```python
from build123d import *

# Parameters (mm, degrees)
BOSS_EXTRUDE1_DEPTH      = 2.38125
BOSS_EXTRUDE1_DEPTH_BACK = 2.38125
SKETCH3_R                = 3.175
SKETCH3_R_2              = 1.4605
CHAMFER1_SIZE            = 0.17145
CUT_EXTRUDE1_DEPTH       = 6.082479863
CUT_EXTRUDE1_DEPTH_BACK  = 6.082479863
SKETCH4_R                = 1.6002


with BuildPart() as part:
    # Sketch3 → Boss-Extrude1 (new, two sides: drawn at the far end of the back side and taken through both)
    with BuildSketch(Plane.XY.offset(-BOSS_EXTRUDE1_DEPTH_BACK)):
        Circle(SKETCH3_R)
        Circle(SKETCH3_R_2, mode=Mode.SUBTRACT)
    extrude(amount=BOSS_EXTRUDE1_DEPTH + BOSS_EXTRUDE1_DEPTH_BACK)

    # Chamfer1
    chamfer1_edges = [part.edges().sort_by_distance(p)[0] for p in [
        (-3.175, 0, -2.38125),
        (-1.4605, 0, -2.38125),
        (-3.175, 0, 2.38125),
        (-1.4605, 0, 2.38125),
    ]]
    chamfer(chamfer1_edges, length=CHAMFER1_SIZE)

    # Sketch4 → Cut-Extrude1 (cut, two sides: drawn at the far end of the back side and taken through both)
    with BuildSketch(Plane.XY.offset(-CUT_EXTRUDE1_DEPTH_BACK)):
        Circle(SKETCH4_R)
    extrude(amount=CUT_EXTRUDE1_DEPTH + CUT_EXTRUDE1_DEPTH_BACK, mode=Mode.SUBTRACT)


solid = part.part
```
Here's how the part is built. I have some questions about the finished solid (model axes, mm). Round coordinates to 2 decimals unless told otherwise and drop trailing zeros. Order: outer loops, then holes, each group sorted by start corner. A loop starts at its lowest first (then second) coordinate and runs counter-clockwise, first axis right, second up. Notation, with made-up numbers: (81.5, 72.25) -> (96.5, 72.25) arc R34 cw to (96.5, 104.25) -> close; hole circle Ø10 at (47.5, 69.5). An arc over 180 degrees is marked (long way). Use a Markdown table: item, result. Add a question column.
(1) I need wall thicknesses on line 1 along Y through (x, z) = (0, -0.65) (3 decimals); line 2 along Y through (x, z) = (1, 2.1); line 3 along X through (y, z) = (0.75, 1.25). Which ranges of each line are inside material? Lowest first, please.
(2) If we mould it in two halves opening along Y, with no side actions, what happens to faces 1 (the face through (1.3, -1.3, -2.381)), 2 (the face through (-1.27, -0.974, -0.033)), 3 (the face through (-0.69, -3.1, -0.03))? For each: released by +Y, released by -Y, zero draft, split by the parting line, or undercut.
(3) Suppose I cut it at C-C, the plane z = -2. Please give me the cut outline in (x, y) (3 decimals), and give its area (3 significant figures).
(4) For pin 1 Ø1.5 at (y, z) = (-1, 0.5) entering from +X; pin 2 Ø2.5 at (x, y) = (0, 0) entering from +Z, each with a flat end and sliding along its axis, tell me the tip position at first contact or that it passes through.
Verdict:
| question | item | result |
|---|---|---|
| 1 | line 1 | -3.175 to -1.6, 1.6 to 3.175 |
| 1 | line 2 | -3.01 to -1.25, 1.25 to 3.01 |
| 1 | line 3 | -3.09 to -1.41, 1.41 to 3.09 |
| 2 | face 1 | zero draft |
| 2 | face 2 | undercut |
| 2 | face 3 | split by the parting line |
| 3 | outline | circle Ø6.35 at (0, 0); hole circle Ø3.2 at (0, 0) |
| 3 | area | 23.6 mm2 |
| 4 | pin 1 | x = 3.17 |
| 4 | pin 2 | through |
